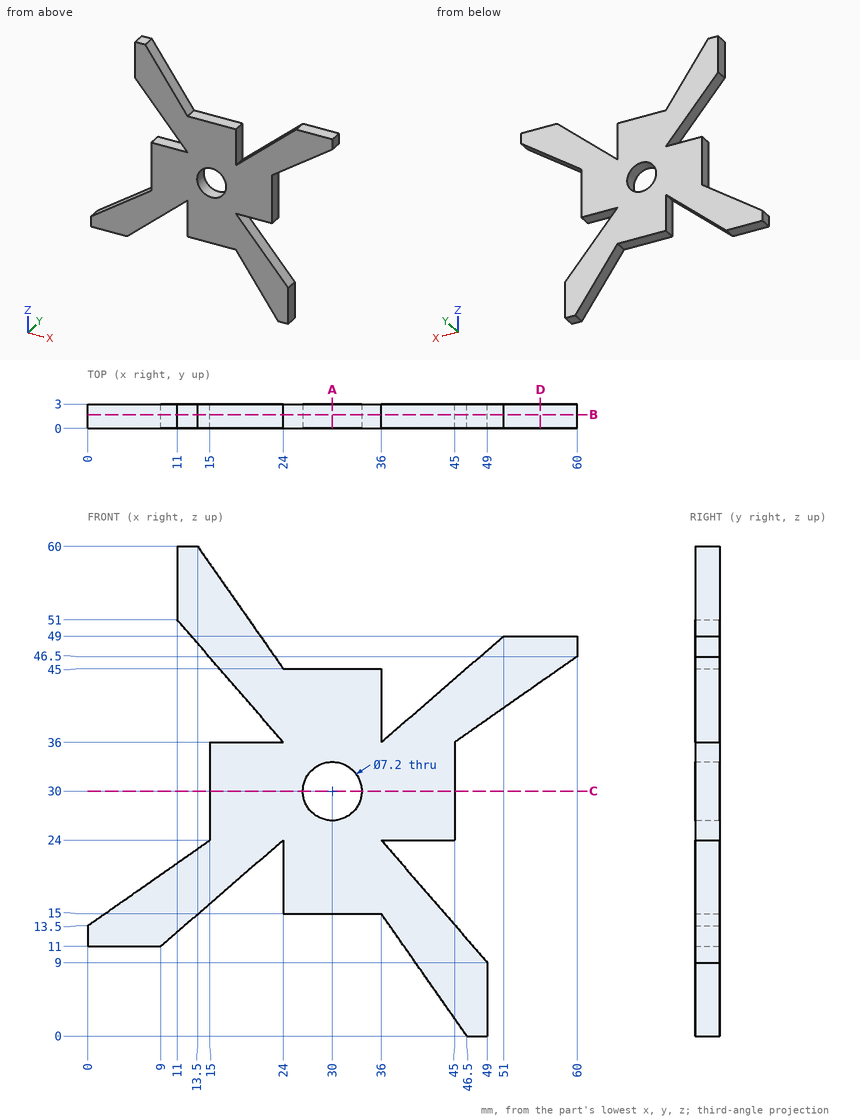
Part print with two shaded views. Sizes in mm from the minimum x, y, z corner. Coordinates: 2 decimals unless noted, no trailing zeros. Loops run counter-clockwise (first coordinate to the right, second up) from the corner with the lowest first, then second, coordinate; pieces in that order, holes last. Notation, with made-up numbers: M 16.5,30.5 L 55.5,30.5 A10 cw 55.5,47.5 Z; hole C 18.5,-6 d3. An arc over 180 degrees is marked long. Use CSV: the item, a comma, the result in double quotes. Start each with the question number.
1. Band-saw the part on D-D, the plane x = 55.5. List the corners of the cut face in (y, z).
2. Band-saw the part on C-C, the plane z = 30. List the corners of the cut face in (x, y).
3. Band-saw the part on B-B, the plane y = 1.7. List the corners of the cut face in (x, z), then the cut area to 3 significant figures.
4. Band-saw the part on A-A, the plane x = 30. List the corners of the cut face in (y, z).
5. Flat gauge pins, fed straight in: pin 1 (1.5 mm diameter, centred on x = 31, y = 2, fed in from -Z); pin 2 (0.9 mm diameter, centred on y = 1, z = 40.5, fed in from +X); pin 3 (1.5 mm diameter, centred on x = 38.5, y = 1.5, fed in from -Z). Where does each tip first touch, or does it go through?
6. Probe probe 1 along X at (y, z) = (0.75, 30); probe 2 along X at (y, z) = (2.5, 25); probe 3 along X at (y, z) = (1.65, 17). List the from-to ranges inside material, lowest first. Write a range as [from, to].
Entries:
1,outline,"M 0,43.35 L 3,43.35 L 3,49 L 0,49 Z"
2,outline,"M 15,0 L 26.4,0 L 26.4,3 L 15,3 Z; M 33.6,0 L 45,0 L 45,3 L 33.6,3 Z"
3,outline,"M 0,11 L 9,11 L 24,24 L 24,15 L 36,15 L 46.5,0 L 49,0 L 49,9 L 36,24 L 45,24 L 45,36 L 60,46.5 L 60,49 L 51,49 L 36,36 L 36,45 L 24,45 L 13.5,60 L 11,60 L 11,51 L 24,36 L 15,36 L 15,24 L 0,13.5 Z; hole C 30,30 d7.2"
3,area,"1,080 mm2"
4,outline,"M 0,15 L 3,15 L 3,26.4 L 0,26.4 Z; M 0,33.6 L 3,33.6 L 3,45 L 0,45 Z"
5,pin 1,"stops at z = 15"
5,pin 2,"stops at x = 52.07"
5,pin 3,"stops at z = 10.36"
6,probe 1,"x = [15, 26.4], [33.6, 45]"
6,probe 2,"x = [15, 45]"
6,probe 3,"x = [5, 15.92], [24, 42.07]"
